Autodesk Fusion 360 part; units mm, degrees
sketch "Sketch1" plane through (0, 0, 0) normal (0, 0, 1) x (1, 0, 0)
  line L0 (0.5, 0) -> (51.2, 0)
  line L1 (51.7, 0.5) -> (51.7, 32.2)
  line L2 (51.2, 32.7) -> (0.5, 32.7)
  line L3 (0, 32.2) -> (0, 0.5)
  line L4 (51.7, 32.7) -> (0, 0) construction
  line L5 (0, 32.7) -> (51.7, 0) construction
  line L6 (51.7, 16.35) -> (0, 16.35) construction
  line L7 (25.85, 32.7) -> (25.85, 0) construction
  line L8 (51.7, 16.35) -> (48.35, 16.35) construction
  line L9 (0, 16.35) -> (3.35, 16.35) construction
  line L10 (25.85, 0) -> (25.85, 3) construction
  line L11 (25.85, 3) -> (48.2, 3) construction
  line L12 (25.85, 3) -> (0, 3) construction
  line L13 (25.85, 32.7) -> (25.85, 28.35) construction
  line L14 (25.85, 28.35) -> (51.7, 28.35) construction
  line L15 (25.85, 28.35) -> (0, 28.35) construction
  line L16 (3.5, 28.35) -> (48.2, 28.35)
  line L17 (48.7, 27.85) -> (48.7, 3.5)
  line L18 (48.7, 3) -> (3.5, 3)
  line L19 (3, 3.5) -> (3, 27.85)
  arc A0 (0.5, 32.7) -> (0, 32.2) centre (0.5, 32.2) ccw
  arc A1 (3.5, 28.35) -> (3, 27.85) centre (3.5, 27.85) ccw
  arc A2 (3, 3.5) -> (3.5, 3) centre (3.5, 3.5) ccw
  arc A3 (0, 0.5) -> (0.5, 0) centre (0.5, 0.5) ccw
  arc A4 (51.2, 0) -> (51.7, 0.5) centre (51.2, 0.5) ccw
  arc A5 (51.7, 32.2) -> (51.2, 32.7) centre (51.2, 32.2) ccw
  arc A6 (48.7, 27.85) -> (48.2, 28.35) centre (48.2, 27.85) ccw
  arc A7 (48.2, 3) -> (48.7, 3.5) centre (48.2, 3.5) ccw
  point P0 (25.85, 16.35)
  point P1 (48.35, 32.7)
  point P2 (48.35, 0)
  dimension "d1" = 51.7
  dimension "d2" = 32.7
  dimension "d5" = 3
  dimension "d6" = 4.35
  dimension "d7" = 0.5
  dimension "d8" = 0.5
  dimension "d9" = 0.5
  dimension "d10" = 0.5
  dimension "d11" = 0.5
  dimension "d12" = 0.5
  dimension "d13" = 0.5
  dimension "d14" = 0.5
  dimension "d32" = 3
  dimension "d33" = 3
extrude "Extrude1" add sketch "Sketch1" along normal blind 5
sketch "Sketch2" plane through (0, 0, 5) normal (0, 0, 1) x (-1, 0, 0)
  arc A0 (-3, -3.5) -> (-3.5, -3) centre (-3.5, -3.5) ccw
  line L0 (-3, -3.5) -> (-3, -27.85)
  arc A1 (-3.5, -28.35) -> (-3, -27.85) centre (-3.5, -27.85) ccw
  line L1 (-3.5, -28.35) -> (-48.2, -28.35)
  arc A2 (-48.7, -27.85) -> (-48.2, -28.35) centre (-48.2, -27.85) ccw
  line L2 (-48.7, -27.85) -> (-48.7, -3.5)
  arc A3 (-48.2, -3) -> (-48.7, -3.5) centre (-48.2, -3.5) ccw
  line L3 (-48.2, -3) -> (-3.5, -3)
  arc A4 (-51.7, -32.2) -> (-51.2, -32.7) centre (-51.2, -32.2) ccw
  line L4 (-51.2, -32.7) -> (-0.5, -32.7)
  arc A5 (-0.5, -32.7) -> (0, -32.2) centre (-0.5, -32.2) ccw
  line L5 (0, -32.2) -> (0, -0.5)
  arc A6 (0, -0.5) -> (-0.5, 0) centre (-0.5, -0.5) ccw
  line L6 (-0.5, 0) -> (-51.2, 0)
  arc A7 (-51.2, 0) -> (-51.7, -0.5) centre (-51.2, -0.5) ccw
  line L7 (-51.7, -0.5) -> (-51.7, -32.2)
  line L8 (-51.7, -28.35) -> (0, -28.35) construction
  line L9 (-11.35, -32.7) -> (-40.35, -32.7)
  line L10 (-40.85, -32.2) -> (-40.85, -28.85)
  line L11 (-40.35, -28.35) -> (-11.35, -28.35)
  line L12 (-10.85, -28.85) -> (-10.85, -32.2)
  arc A8 (-11.35, -32.7) -> (-10.85, -32.2) centre (-11.35, -32.2) ccw
  arc A9 (-10.85, -28.85) -> (-11.35, -28.35) centre (-11.35, -28.85) ccw
  arc A10 (-40.85, -32.2) -> (-40.35, -32.7) centre (-40.35, -32.2) ccw
  arc A11 (-40.35, -28.35) -> (-40.85, -28.85) centre (-40.35, -28.85) ccw
  point P0 (-10.85, -32.7)
  point P1 (-40.85, -32.7)
  point P2 (-10.85, -32.7)
  point P3 (-40.85, -32.7)
  point P4 (-10.85, -28.35)
  dimension "d19" = 4.35
  dimension "d20" = 30
  dimension "d21" = 4.35
  dimension "d22" = 0.5
  dimension "d23" = 0.5
  dimension "d24" = 0.5
  dimension "d25" = 0.5
extrude "Extrude2" add sketch "Sketch2" along normal blind 5 contours L1 L4 L9 L10 L11 L12 A8 A9 A10 A11
sketch "Sketch3" plane through (40.85, 0, 0) normal (1, 0, 0) x (0, 1, 0)
  line L0 (28.85, 5) -> (32.2, 5)
  line L1 (32.2, 5) -> (32.2, 10)
  line L2 (32.2, 10) -> (28.85, 10)
  line L3 (28.85, 10) -> (28.85, 5)
  line L4 (28.85, 10) -> (32.2, 5) construction
  line L5 (32.2, 10) -> (28.85, 5) construction
  line L6 (32.2, 7.5) -> (28.85, 7.5) construction
  circle A0 centre (30.525, 7.5) radius 0.8
  point P0 (30.525, 7.5)
  dimension "d28" = 1.6
extrude "Extrude3" cut sketch "Sketch3" against normal blind 40 contours A0
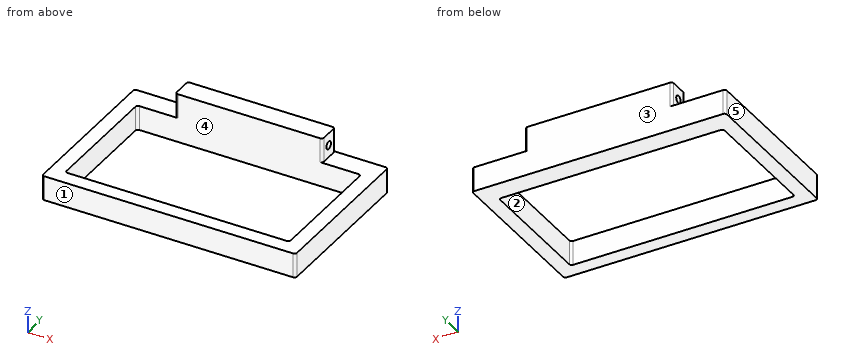
Geometry: final body of the model. Coordinates: model frame, mm. Face numbers are marked on the shaded views. A direction names the side the tool comes from. Coordinates: 2 decimals unless noted, no trailing zeros. Order: outer loops, then holes, each group sorted by start corner. A loop starts at its lowest first (then second) coordinate and runs counter-clockwise, first axis right, second up. Notation, with made-up numbers: (30.5, -22.5) -> (60.5, -22.5) arc R20 ccw to (60.5, -13.5) -> close; hole circle Ø4 at (-12.75, -37.75). An arc over 180 degrees is marked (long way). Write each question's results on one line, items separated by ' | '. Start each with the question number.
1) Mould query, pull axis Y, two halves, no side actions, for the marked faces 3, 4 and 5. Classes: released by +Y, released by -Y, zero draft, split by the parting line, or undercut.
2) Material intervals for line 1 along X through (y, z) = (15, 3.5); line 2 along Y through (x, z) = (46.5, 2.25); line 3 along Z through (x, y) = (48, 30), sorted ascending.
3) First-contact query: pin 1 (2 mm diameter, centred on y = 30.525, z = 7.5, fed in from -X); pin 2 (5 mm diameter, centred on x = 16.5, z = 3, fed in from -Y); pin 3 (6 mm diameter, centred on x = 14.5, y = 6.5, fed in from +Z); pin 4 (16.5 mm diameter, centred on x = 21.5, y = 9, fed in from +Z). Flat tips, straight axial feed; report the tip coordinate or a pass-through.
4) Cut plane A-A, the plane x = 20. Output: boundary loops of the cut face in (y, z) (3 decimals), and give its area (3 significant figures).
5) Cut plane D-D, the plane y = 30.5. Output: boundary loops of the cut face in (x, z).
6) Set-up query: the marked faces 1 and 2. Return all of +Z, -Z, +X, -X, +Y, -Y with unobstructed straight access to the full face (end or side cutting, diameter ignored); none if empty.
7) Cut plane C-C, the plane z = 7.5. Output: boundary loops of the cut face in (x, y) (3 decimals), and give its area (3 significant figures).
8) Cut plane B-B, the plane x = 46.5. Output: boundary loops of the cut face in (y, z).
Checks:
1) face 3: released by +Y | face 4: undercut | face 5: zero draft
2) line 1: 0 to 3, 48.7 to 51.7 | line 2: 0 to 3, 28.35 to 32.7 | line 3: 0 to 5
3) pin 1: x = 10.85 | pin 2: y = 0 | pin 3: through | pin 4: z = 5
4) outline: (0, 0) -> (3, 0) -> (3, 5) -> (0, 5) -> close; (28.35, 0) -> (32.7, 0) -> (32.7, 10) -> (28.35, 10) -> close; hole circle Ø1.6 at (30.525, 7.5) | area: 56.5 mm^2
5) outline: (0, 0) -> (51.7, 0) -> (51.7, 5) -> (40.85, 5) -> (40.85, 6.7) -> (10.85, 6.7) -> (10.85, 5) -> (0, 5) -> close; (10.85, 8.3) -> (40.85, 8.3) -> (40.85, 10) -> (10.85, 10) -> close
6) face 1: +Z, -Z, +X, -X, -Y | face 2: +Z, -Z
7) outline: (10.85, 28.85) arc R0.5 ccw to (11.35, 28.35) -> (40.35, 28.35) arc R0.5 ccw to (40.85, 28.85) -> (40.85, 29.725) -> (10.85, 29.725) -> close; (10.85, 31.325) -> (40.85, 31.325) -> (40.85, 32.2) arc R0.5 ccw to (40.35, 32.7) -> (11.35, 32.7) arc R0.5 ccw to (10.85, 32.2) -> close | area: 82.3 mm^2
8) outline: (0, 0) -> (3, 0) -> (3, 5) -> (0, 5) -> close; (28.35, 0) -> (32.7, 0) -> (32.7, 5) -> (28.35, 5) -> close
